from build123d import *

# Parameters (mm, degrees)
CROQUIS1_R              = 2.35
CROQUIS1_R_2            = 2.225
SALIENTE_EXTRUIR1_DEPTH = 7.25
SALIENTE_EXTRUIR2_START = 7.25
CROQUIS1_3_R            = 2.225
SALIENTE_EXTRUIR2_DEPTH = 20
CORTAR_EXTRUIR1_START   = -6.5
CORTAR_EXTRUIR1_DEPTH   = 6.5


with BuildPart() as part:
    # Croquis1 → Saliente-Extruir1 (new body)
    # profile 1 of 2: a face of its own
    with BuildSketch(Plane.YZ):
        with Locations(Location((0, 0, 0), (0, 0, 90))):
            Circle(CROQUIS1_R)
        Circle(CROQUIS1_R_2, mode=Mode.SUBTRACT)
    # profile 2 of 2: a face of its own
    with BuildSketch(Plane.YZ):
        Circle(CROQUIS1_R_2)
    extrude(amount=SALIENTE_EXTRUIR1_DEPTH)

    # Croquis1<3> → Saliente-Extruir2 (add)
    with BuildSketch(Plane.YZ.offset(SALIENTE_EXTRUIR2_START)):
        with Locations(Location((0, 0, 0), (0, 0, 270))):
            Circle(CROQUIS1_3_R)
    extrude(amount=SALIENTE_EXTRUIR2_DEPTH)

    # Croquis3 → Cortar-Extruir1 (cut)
    with BuildSketch(Plane.YZ.offset(27.25).offset(CORTAR_EXTRUIR1_START)):
        with BuildLine():
            ThreePointArc((1.573312588, 1.573312588), (0, 2.225), (-1.573312588, 1.573312588))
            Line((-1.573312588, 1.573312588), (1.573312588, 1.573312588))
        make_face()
        with BuildLine():
            ThreePointArc((-1.573312588, 1.573312588), (-2.225, 0), (-1.573312588, -1.573312588))
            Line((-1.573312588, -1.573312588), (-1.573312588, 1.573312588))
        make_face()
        with BuildLine():
            Line((1.573312588, 1.573312588), (1.573312588, -1.573312588))
            ThreePointArc((1.573312588, -1.573312588), (2.05563196, -0.851470637), (2.225, 0))
            ThreePointArc((2.225, 0), (2.05563196, 0.851470637), (1.573312588, 1.573312588))
        make_face()
        with BuildLine():
            Line((1.573312588, -1.573312588), (-1.573312588, -1.573312588))
            ThreePointArc((-1.573312588, -1.573312588), (0, -2.225), (1.573312588, -1.573312588))
        make_face()
    extrude(amount=CORTAR_EXTRUIR1_DEPTH, mode=Mode.SUBTRACT)


solid = part.part
Can you work these out from the model? Positions are in its coordinate system, mm. A direction names the side the tool comes from. Coordinates: 2 decimals unless noted, no trailing zeros. Write each loop counter-clockwise with the first axis right and the second up, starting at its lowest first coordinate (ties: lowest second). Pieces come first, ordered by that corner, then holes. Notation, with made-up numbers: (84, 8) -> (101, 8) arc R29 ccw to (101, 29) -> close; hole circle Ø8 at (36, 84.25). An arc over 180 degrees is marked (long way). Answer as CSV lines item,"result".
1) Will these pins go through, and if not, where does the flat tip stop? P1, Ø1, axis at x = 10, y = 0.5, coming from the +Z side (3 decimals); P2, Ø1.6, axis at x = 22.5, y = 0.5, coming from the +Z side; P3, Ø0.5, axis at y = -2, z = 0.5, coming from the +X side.
Check result:
P1,"z = 2.225"
P2,"z = 1.57"
P3,"x = 20.75"
2) If we section it at A-A on z = 0: Please give me the cut outline in (x, y) (3 decimals), then the cut area to 3 significant figures.
Check result:
outline,"(0, -2.35) -> (7.25, -2.35) -> (7.25, -2.225) -> (20.75, -2.225) -> (20.75, -1.573) -> (27.25, -1.573) -> (27.25, 1.573) -> (20.75, 1.573) -> (20.75, 2.225) -> (7.25, 2.225) -> (7.25, 2.35) -> (0, 2.35) -> close"
area,"115 mm²"
3) If we section it at C-C on x = 2: Please give me the cut outline in (y, z).
Check result:
outline,"circle Ø4.7 at (0, 0)"
4) On a 3-axis mill with a long thin cutter (end or side, diameter ignored), from which of +Z, -Z, +X, -X, +Y, -Y can I reach the whole of each face in a straight line? I mean faces 1 (the flat face through (24, -1.573, 0)), 2 (the flat face through (24, 1.573, 0)), 3 (the flat face through (24, 0, -1.573)). Say none if no direction works.
Check result:
face 1,"+Z, -Z, +X, -Y"
face 2,"+Z, -Z, +X, +Y"
face 3,"-Z, +X, +Y, -Y"
5) If I drill on line 1 (Z direction, x = 25.75, y = -0.7); line 2 (X direction, y = 0.5, z = -2.05); line 3 (Y direction, x = 20.5, z = 0) (3 decimals), over which ranges is the centre line in solid material (lowest first)? Write a range as from..to.
Check result:
line 1,"-1.57..1.57"
line 2,"0..20.75"
line 3,"-2.225..2.225"
6) If we section it at D-D on y = 1.8: Please give me the cut outline in (x, z).
Check result:
outline,"(0, -1.51) -> (7.25, -1.51) -> (7.25, -1.31) -> (20.75, -1.31) -> (20.75, 1.31) -> (7.25, 1.31) -> (7.25, 1.51) -> (0, 1.51) -> close"
